The model under review builds one solid part; all positions refer to its coordinate system, in mm. A direction names the side the tool comes from. Round coordinates to 2 decimals unless told otherwise and drop trailing zeros. Loops run counter-clockwise (first coordinate to the right, second up) from the corner with the lowest first, then second, coordinate; pieces in that order, holes last. Notation, with made-up numbers: (16, -16) -> (61, -16) arc R23 ccw to (61, 23) -> close; hole circle Ø3 at (-10.5, 79.25). An arc over 180 degrees is marked (long way). Return JSON: item names as keys, results as strings. Group by question number.
```python
from build123d import *

# Parameters (mm, degrees)
SKETCH1_W           = 139.5
SKETCH1_H           = 152.4
BOSS_EXTRUDE1_DEPTH = 6.35
SKETCH2_W           = 139.5
SKETCH2_H           = 152.4
CUT_EXTRUDE1_DEPTH  = 3.375
SKETCH3_R           = 2.286
BOSS_EXTRUDE2_DEPTH = 12.7
SKETCH4_R           = 2.286
BOSS_EXTRUDE3_DEPTH = 12.7
BOSS_EXTRUDE4_DEPTH = 12.7
CHAMFER1_SIZE       = 1.27
SKETCH6_W           = 8.89
SKETCH6_H           = 2.54
CUT_EXTRUDE2_DEPTH  = 207.995893689


with BuildPart() as part:
    # Sketch1 → Boss-Extrude1 (new body)
    with BuildSketch(Plane(origin=(0, 0, 0), x_dir=(1, 0, 0), z_dir=(0, 1, 0))):
        with Locations((69.75, 76.2)):
            Rectangle(SKETCH1_W, SKETCH1_H)
    extrude(amount=BOSS_EXTRUDE1_DEPTH)

    # Sketch2 → Cut-Extrude1 (cut)
    with BuildSketch(Plane(origin=(0, 6.35, 0), x_dir=(1, 0, 0), z_dir=(0, 1, 0))):
        with Locations((69.75, 76.2)):
            Rectangle(SKETCH2_W, SKETCH2_H)
    extrude(amount=-CUT_EXTRUDE1_DEPTH, mode=Mode.SUBTRACT)

    # Sketch3 → Boss-Extrude2 (add)
    with BuildSketch(Plane.XY):
        with BuildLine():
            Line((63.4, 9.325), (63.4, 2.975))
            Line((63.4, 2.975), (76.1, 2.975))
            Line((76.1, 2.975), (76.1, 9.325000158))
            ThreePointArc((76.1, 9.325000158), (69.749999921, 15.675000158), (63.4, 9.325))
        make_face()
        with Locations((69.75, 9.325000158)):
            Circle(SKETCH3_R, mode=Mode.SUBTRACT)
    extrude(amount=-BOSS_EXTRUDE2_DEPTH)

    # Sketch4 → Boss-Extrude3 (add)
    # profile 1 of 2: a face of its own
    with BuildSketch(Plane(origin=(0, 0, -152.4), x_dir=(-1, 0, 0), z_dir=(0, 0, -1))):
        with BuildLine():
            Line((-130.61, 9.325), (-130.61, 2.975))
            Line((-130.61, 2.975), (-117.91, 2.975))
            Line((-117.91, 2.975), (-117.91, 9.325))
            ThreePointArc((-117.91, 9.325), (-124.26, 15.675), (-130.61, 9.325))
        make_face()
        with Locations((-124.26, 9.325)):
            Circle(SKETCH4_R, mode=Mode.SUBTRACT)
    # profile 2 of 2: a face of its own
    with BuildSketch(Plane(origin=(0, 0, -152.4), x_dir=(-1, 0, 0), z_dir=(0, 0, -1))):
        with BuildLine():
            Line((-21.59, 9.325), (-21.59, 2.975))
            Line((-21.59, 2.975), (-8.89, 2.975))
            Line((-8.89, 2.975), (-8.89, 9.325))
            ThreePointArc((-8.89, 9.325), (-15.24, 15.675), (-21.59, 9.325))
        make_face()
        with Locations((-15.24, 9.325)):
            Circle(SKETCH4_R, mode=Mode.SUBTRACT)
    extrude(amount=-BOSS_EXTRUDE3_DEPTH)

    # Sketch5 → Boss-Extrude4 (add)
    with BuildSketch(Plane(origin=(0, 2.975, 0), x_dir=(1, 0, 0), z_dir=(0, 1, 0))):
        Polygon((36.73, 146.05), (36.73, 133.35), (39.27, 133.35), (39.27, 143.51), (100.23, 143.51), (100.23, 133.35), (102.77, 133.35), (102.77, 146.05), align=None)
        Polygon((39.27, 104.14), (100.23, 104.14), (100.23, 114.3), (102.77, 114.3), (102.77, 101.6), (36.73, 101.6), (36.73, 114.3), (39.27, 114.3), align=None)
    extrude(amount=BOSS_EXTRUDE4_DEPTH)

    # Chamfer1
    chamfer1_edges = [part.edges().sort_by_distance(p)[0] for p in [
        (100.23, 15.675, -109.22),
        (69.75, 15.675, -104.14),
        (39.27, 15.675, -109.22),
        (38, 15.675, -114.3),
        (36.73, 15.675, -107.95),
        (69.75, 15.675, -101.6),
        (102.77, 15.675, -107.95),
        (101.5, 15.675, -114.3),
        (39.27, 15.675, -138.43),
        (69.75, 15.675, -143.51),
        (100.23, 15.675, -138.43),
        (101.5, 15.675, -133.35),
        (102.77, 15.675, -139.7),
        (69.75, 15.675, -146.05),
        (36.73, 15.675, -139.7),
        (38, 15.675, -133.35),
    ]]
    chamfer(chamfer1_edges, length=CHAMFER1_SIZE - 0.0001)  # a hair under: the kernel refuses the full size

    # Sketch6 → Cut-Extrude2 (cut, through all)
    with BuildSketch(Plane(origin=(0, 2.975, 0), x_dir=(1, 0, 0), z_dir=(0, 1, 0))):
        with Locations((48.795, 147.32)):
            Rectangle(SKETCH6_W, SKETCH6_H)
        with Locations((90.705, 147.32)):
            Rectangle(SKETCH6_W, SKETCH6_H)
        with Locations((48.795, 100.33)):
            Rectangle(SKETCH6_W, SKETCH6_H)
        with Locations((90.705, 100.33)):
            Rectangle(SKETCH6_W, SKETCH6_H)
    extrude(amount=-CUT_EXTRUDE2_DEPTH, mode=Mode.SUBTRACT)


solid = part.part
```
1. We need section A-A, the plane x = 124.26. Write out the cut boundary in (y, z) (3 decimals).
2. Draft analysis for pull direction Y (two halves, no side actions). For faces 5 (the face through (21.59, 6, -146)), 6 (the face through (124.12, 15.673, -146.139)), 7 (the face through (13.13, 8.45, -146.14)), state which applies: pulls with the +Y half, pulls with the -Y half, needs draft (parallel to the pull), parting line crosses it, or undercut.
3. Wall thickness on line 1 (Z direction, x = 66, y = 5); line 2 (Z direction, x = 42, y = 3.75); line 3 (Y direction, x = 124, z = -148): over which ranges is each line inside the solid? List them lowest first.
4. For P1, Ø3, axis at x = 102, y = 9, coming from the +Z side; P2, Ø6, axis at x = 46, z = -127.5, coming from the +Y side (3 decimals); P3, Ø2.5, axis at x = 15.24, y = 9.325, coming from the +Z side; P4, Ø5.5, axis at x = 69.75, y = 9.325, coming from the -Z side, all flat-tipped, find the tip position at first contact; note any pin that passes through.
5. We need section B-B, the plane x = 51. Give the number of separate pieces and of enclosed holes in the cut face, then the cut area to 3 significant figures.
6. Tool access review of faces 1 (the face through (39.27, 9, -109)), 2 (the face through (117.91, 6, -146)), 3 (the face through (36.73, 9, -108)), 4 (the face through (15.3, 6.6, -139.7)): name each direction out of +Z, -Z, +X, -X, +Y, -Y from which nothing blocks a thin tool from reaching the whole face with its end or side.
Check sheet entries:
{
 "1": {"outline": "(0, -152.4) -> (7.039, -152.4) -> (7.039, -139.7) -> (2.975, -139.7) -> (2.975, 0) -> (0, 0) -> close; (11.611, -152.4) -> (15.675, -152.4) -> (15.675, -139.7) -> (11.611, -139.7) -> close"},
 "2": {"face 5": "needs draft", "face 6": "pulls with the +Y half", "face 7": "undercut"},
 "3": {"line 1": "z = -146.05 to -143.51, -104.14 to -101.6, -12.7 to 0", "line 2": "z = -146.05 to -143.51, -104.14 to -101.6", "line 3": "y = 0 to 7.05, 11.6 to 15.67"},
 "4": {"P1": "stops at z = -101.6", "P2": "stops at y = 2.975", "P3": "passes through", "P4": "stops at z = -146.05"},
 "5": {"separate pieces": "3", "enclosed holes": "0", "area": "500 mm²"},
 "6": {"face 1": "+Y", "face 2": "+Z, -Z, +Y", "face 3": "+Z, -Z, -X, +Y", "face 4": "+Z, -X, +Y"}
}
